The figure shows three views and two pictorial views of one solid part (mm, origin at its lowest corner). Answer the questions. Coordinates: 2 decimals unless noted, no trailing zeros. Order: outer loops, then holes, each group sorted by start corner. A loop starts at its lowest first (then second) coordinate and runs counter-clockwise, first axis right, second up. Notation, with made-up numbers: (68, 63.25) -> (106, 63.25) arc R22 ccw to (106, 73.25) -> close; hole circle Ø11 at (32, -25.5). An arc over 180 degrees is marked (long way). Use one line per item in the form item = value.
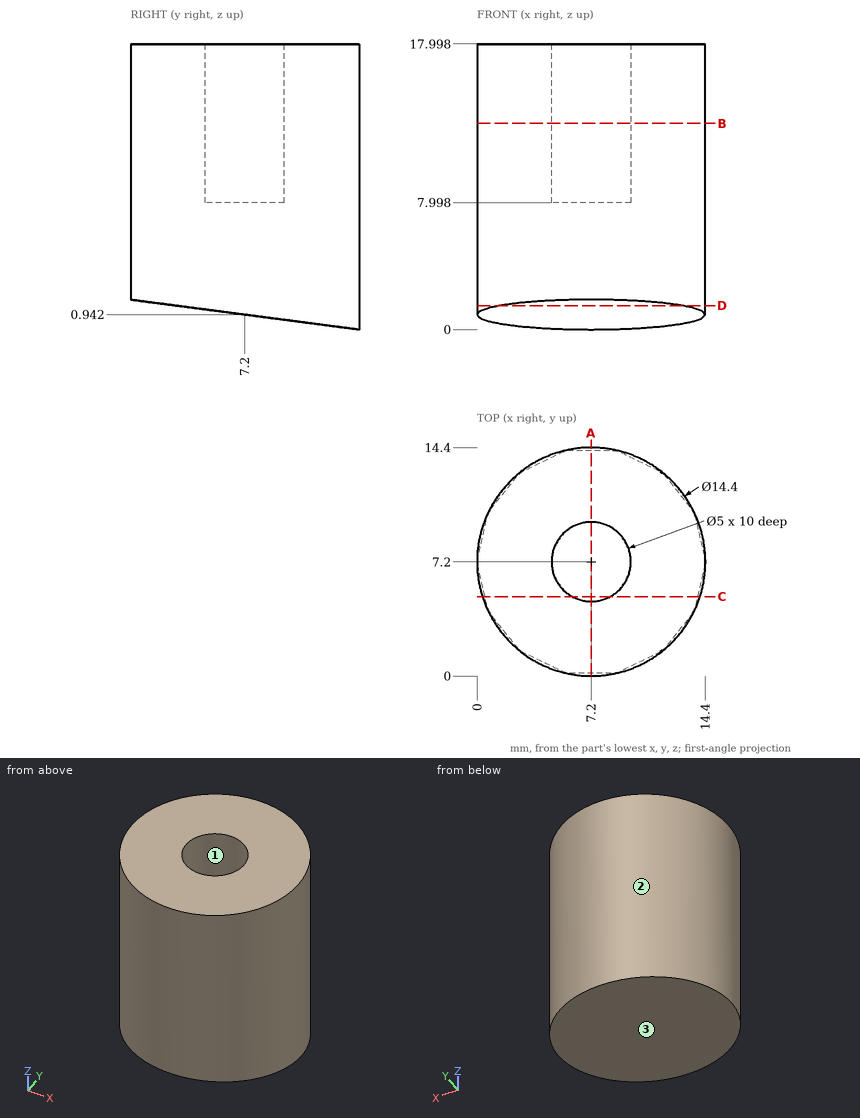
(1) Section A-A on x = 7.2 is taken. Write down the section's boundary in (y, z).
Data:
outline = (0, 1.88) -> (14.4, 0) -> (14.4, 18) -> (9.7, 18) -> (9.7, 8) -> (4.7, 8) -> (4.7, 18) -> (0, 18) -> close
(2) Each of these flat-tipped pins is pushed along its axis until it touches: P1, Ø1.5, axis at x = 11.5, z = 8.5, coming from the +Y side; P2, Ø8, axis at x = 12, z = 12.5, coming from the -Y side; P3, Ø4, axis at x = 7.2, y = 7.2, coming from the -Z side. Where does it stop, or does it pass through?
Data:
P1 = 13.46
P2 = 0.04
P3 = 0.68
(3) Straight lines are drawn through the part: line 1 along Y through (x, z) = (7.2, 13); line 2 along X through (y, z) = (7.75, 12.5); line 3 along X through (y, z) = (8.75, 14.25). For each, find the intervals that lie inside material, in ascending order.
Data:
line_1 = 0 to 4.7, 9.7 to 14.4
line_2 = 0.02 to 4.76, 9.64 to 14.38
line_3 = 0.17 to 5.24, 9.16 to 14.23
(4) Section B-B on z = 13 is taken. Write down the section's boundary in (x, y), plus the area to 3 significant figures.
Data:
outline = circle Ø14.4 at (7.2, 7.2); hole circle Ø5 at (7.2, 7.2)
area = 143 mm²
(5) Section C-C on y = 5 is taken. Write down the section's boundary in (x, z), plus the area to 3 significant figures.
Data:
outline = (0.34, 1.23) -> (14.06, 1.23) -> (14.06, 18) -> (8.39, 18) -> (8.39, 8) -> (6.01, 8) -> (6.01, 18) -> (0.34, 18) -> close
area = 206 mm²
(6) The mould has two halves that part along X. Classify the marked faces 1, 2 and 3: released by +X, released by -X, zero draft, split by the parting line, or undercut.
Data:
face_1 = undercut
face_2 = split by the parting line
face_3 = zero draft
(7) Section D-D on z = 1.5 is taken. Write down the section's boundary in (x, y).
Data:
outline = (1.4, 2.93) -> (13, 2.93) arc R7.2 ccw (long way) to start
